Autodesk Inventor part; units mm, degrees
ref_plane "Work Plane1" through (29, 0, 0) normal (0, -1, 0) x (1, 0, 0)
ref_plane "YZ Plane" through (0, 0, 0) normal (1, 0, 0) x (0, 1, 0)
ref_plane "XZ Plane" through (0, 0, 0) normal (0, 1, 0) x (-1, 0, 0)
sketch "Sketch1" plane through (0, 0, 0) normal (0, 0, 1) x (1, 0, 0)
  line L0 (0.4667, 0) -> (80, 0)
  line L1 (80, 0) -> (80, 4)
  line L2 (80, 4) -> (58, 4)
  line L3 (58, 4) -> (57.2331, 4)
  line L4 (57.2331, 4) -> (0, 4)
  line L5 (0, 4) -> (0, 6.5)
  line L6 (0, 6.5) -> (-5, 6.5)
  line L7 (-5, 6.5) -> (-5, 2.8868)
  line L8 (-5, 2.8868) -> (-1.2, 2.8868)
  line L9 (-1.2, 2.8868) -> (0.4667, 0)
  line L10 (-22, 0) -> (97, 0)
  line L11 (0, -1.3) -> (0, 7.8)
  line L12 (58, 4) -> (0, 4) construction
  dimension "d1" = 22
  dimension "d2" = 0.7669
  dimension "d3" = 5
  dimension "d4" = 3.8
  dimension "d5" = 60
  dimension "d6" = 8
  dimension "d7" = 8
  dimension "d8" = 5.7735
  dimension "d9" = 13
  dimension "d26" = 80
revolve "Body" add sketch "Sketch1" angle 360 about axis through (0.4667, 0, 0) along (1, 0, 0) contours L9 L11 L4 L3 L2 L1 L0 | L9 L8 L7 L6 L5 L11
sketch "Sketch2" plane through (-5, 0, 0) normal (-1, 0, 0) x (0, 0, 1)
  circle A0 centre (0, 0) radius 2.8868
  line L0 (0, -9.1) -> (0, 9.1)
  line L1 (-9.1, 0) -> (9.1, 0)
  line L2 (2.8868, 0) -> (1.4434, -2.5)
  line L3 (1.4434, -2.5) -> (-1.4434, -2.5)
  line L4 (-1.4434, -2.5) -> (-2.8868, 0)
  line L5 (-2.8868, 0) -> (-1.4434, 2.5)
  line L6 (-1.4434, 2.5) -> (1.4434, 2.5)
  line L7 (1.4434, 2.5) -> (2.8868, 0)
extrude "Slot" add sketch "Sketch2" against normal up to next contours L7 A0 | A0 L2 | L6 L0 A0 | A0 L0 L3 | L0 L6 A0 | A0 L3 L0 | L4 A0 | A0 L5
fillet "Fillet1" radius 0.8 1 edges at (-5, -6.5, 0)
thread "Thread"
chamfer "Chamfer1" distance 0.7668 distance2 0.7668 1 edges at (80, -4, 0) measured on face at (80, -0.998, -1.3105)
ref_plane "Work Plane1" through (29, 0, 0) normal (0, -1, 0) x (1, 0, 0)
fillet "Fillet2" radius 0.1 1 edges at (0, -4, 0)
equation "\"d1\" = GEL"
equation "\"d3\" = KOH"
equation "\"d4\" = INTI"
equation "\"d6\" = GD"
equation "\"d7\" = BDM"
equation "\"d8\" = 1.1547 * SW"
equation "\"d9\" = KOD"
equation "\"d26\" = NLG"
equation "\"d30\" = R"
equation "\"d17\" = RR"
equation "\"d13\" = GEL"
equation "\"d15\" = -0.5 * SPD + 0.5 * GD"
equation "\"d16\" = GUL"
equation "\"GD\" = NND"
equation "\"NLG\" = 80"
equation "\"GEL\" = 22"
equation "\"KOD\" = 13"
equation "\"KOH\" = 5"
equation "\"INTI\" = 3.8"
equation "\"GAL\" = 0.61345 * PTC"
equation "\"GUL\" = 0.61345 * PTC"
equation "\"BDM\" = NND"
equation "\"SW\" = 5"
equation "\"RR\" = 0.8"
equation "\"SPD\" = NND - 1.2269 * PTC"
equation "\"R\" = 0.1"
equation "\"TOA\" = 30deg"
equation "\"GD1\" = THREADDIA - 1.2269 * PTC"
equation "\"THREADDIA\" = 8"
equation "\"FAWI\" = 45deg"
equation "\"ANG\" = 120deg"
equation "\"PTC\" = 1.25"
equation "\"NND\" = 8"
equation "\"E0\" = 1.155 * SW"
properties part number "DIN 7984 - M8 x 80" material "Steel, Mild"
Input: part model. Units: mm. Frame: model coordinates. A direction names the side the tool comes from. Coordinates: 2 decimals unless noted, no trailing zeros. Loops run counter-clockwise (first coordinate to the right, second up) from the corner with the lowest first, then second, coordinate; pieces in that order, holes last. Notation, with made-up numbers: M 58.25,-10.75 L 80.25,-10.75 A19 ccw 80.25,15.25 Z; hole C -34,75.25 d9. An arc over 180 degrees is marked long. Answer in a Markdown table with one row per item.
1. Draft query along Z for faces 1 (the cylindrical face through (39.113, -0.867, 3.905)), 2 (the flat face through (-3.017, -1.268, -2.155)), 3 (the flat face through (80, 0, 0)). Return one class per face: pulls with the +Z half, pulls with the -Z half, needs draft (parallel to the pull), parting line crosses it, or undercut.
Response:
| item | result |
|---|---|
| face 1 | parting line crosses it |
| face 2 | undercut |
| face 3 | needs draft |
2. Reachability of faces 4 (the cylindrical face through (-2.129, -5.158, 3.955)), 5 (the flat face through (0, 1.4, -4.2)), 6 (the flat face through (-3.017, 1.233, -2.175)) from +Z, -Z, +X, -X, +Y, -Y: full face, straight path, thin tool, end or side. Return the list, or none.
Response:
| item | result |
|---|---|
| face 4 | +X, -X |
| face 5 | +X |
| face 6 | -X |
3. Section A-A, the plane x = 40.5. Output: boundary loops of the cut face in (y, z), then the cut area to 3 significant figures.
Response:
| item | result |
|---|---|
| outline | C 0,0 d8 |
| area | 50.3 mm2 |
4. First-contact query: pin 1 (1.5 mm diameter, centred on x = 22, y = 0, fed in from -Z); pin 2 (1 mm diameter, centred on x = 43, z = 0, fed in from -Y); pin 3 (0.9 mm diameter, centred on x = -3.5, z = 0.5, fed in from +Y); pin 4 (3 mm diameter, centred on x = 60.5, y = 4, fed in from +Z). Flat tips, straight axial feed; report the tip coordinate or a pass-through.
Response:
| item | result |
|---|---|
| pin 1 | stops at z = -4 |
| pin 2 | stops at y = -4 |
| pin 3 | stops at y = 6.5 |
| pin 4 | stops at z = 3.12 |
5. Material intervals for line 1 (X direction, y = -3.75, z = -4.25); line 2 (Y direction, x = 68, z = -2.5); line 3 (Z direction, x = 68, y = -1.75), sorted ascending.
Response:
| item | result |
|---|---|
| line 1 | x = -5 to 0 |
| line 2 | y = -3.12 to 3.12 |
| line 3 | z = -3.6 to 3.6 |
